Build history of the part. All positions in model axes, mm. A direction names the side the tool comes from. Give positions to 0.01 mm unless a question says otherwise; leave off trailing zeros. Order: outer loops, then holes, each group sorted by start corner. A loop starts at its lowest first (then second) coordinate and runs counter-clockwise, first axis right, second up. Notation, with made-up numbers: (82, 65.5) - (105, 65.5) arc R24 ccw to (105, 89.5) - close; hole circle Ø11 at (54, 16.25). An arc over 180 degrees is marked (long way). Use a Markdown table: item, result.
Autodesk Inventor part; units mm, degrees
ref_plane "YZ Plane" through (0, 0, 0) normal (1, 0, 0) x (0, 1, 0)
ref_plane "XZ Plane" through (0, 0, 0) normal (0, 1, 0) x (-1, 0, 0)
ref_plane "XY Plane" through (0, 0, 0) normal (0, 0, 1) x (1, 0, 0)
sketch "スケッチ1" plane through (0, 0, 0) normal (0, 0, 1) x (1, 0, 0)
  circle A0 centre (0, 0) radius 12.675
  circle A1 centre (0, 0) radius 4
  circle A2 centre (0, 0) radius 10
  circle A3 centre (0, 0) radius 16
  dimension "d0" = 25.35
  dimension "d1" = 8
  dimension "d2" = 20
  dimension "d3" = 32
extrude "押し出し1" add sketch "スケッチ1" along normal blind 3.75 contours A2
extrude "押し出し2" add sketch "スケッチ1" against normal blind 1.7 contours A0
extrude "押し出し3" add sketch "スケッチ1" against normal blind 2.5 contours A2
mirror "ミラー1" about plane through (0, 0, 3.75) normal (0, 0, 1) of "押し出し1", "押し出し2", "押し出し3"
properties part number "timing _pulley_7.5_8"
1) Slice it at D-D (x = 7). Write the cut outline in (y, z), and give its area (3 significant figures).
Computed:
| item | result |
|---|---|
| outline | (-10.57, -1.7) - (-7.14, -1.7) - (-7.14, -2.5) - (7.14, -2.5) - (7.14, -1.7) - (10.57, -1.7) - (10.57, 0) - (7.14, 0) - (7.14, 7.5) - (10.57, 7.5) - (10.57, 9.2) - (7.14, 9.2) - (7.14, 10) - (-7.14, 10) - (-7.14, 9.2) - (-10.57, 9.2) - (-10.57, 7.5) - (-7.14, 7.5) - (-7.14, 0) - (-10.57, 0) - close |
| area | 202 mm² |
2) Wall check: line 1 (Y direction, x = 0, z = 2.25); line 2 (Z direction, x = 4, y = -10.5); line 3 (X direction, y = 1, z = 5). Give the ranges that are in metal, low to high. Write a range as from..to.
Computed:
| item | result |
|---|---|
| line 1 | y = -10..-4, 4..10 |
| line 2 | z = -1.7..0, 7.5..9.2 |
| line 3 | x = -9.95..-3.87, 3.87..9.95 |
3) Tool access for faces 1 (the flat face through (0.9, 10.4, -1.7)), 2 (the flat face through (0.9, 10.4, 0)), 3 (the cylindrical face through (-2.17, 9.76, 9.59)): list every direction of +Z, -Z, +X, -X, +Y, -Y with a clear straight run to the whole face (end or side of a thin tool).
Computed:
| item | result |
|---|---|
| face 1 | -Z |
| face 2 | none |
| face 3 | +Z |
4) Two-plate mould, pull along Z, no slides. Class faces 4 (the cylindrical face through (-2.17, -9.76, -2.09)), 5 (the flat face through (-4.3, 0.1, 10)), 6 (the cylindrical face through (-2.17, 9.76, 3.7)): +Z half, -Z half, draft (parallel to the pull), parting line (faces both ways), or undercut.
Computed:
| item | result |
|---|---|
| face 4 | draft |
| face 5 | +Z half |
| face 6 | undercut |
5) Pin check, flat tips, straight feed: P1, Ø1.5, axis at y = 0.5, z = 4.5, coming from the +X side; P2, Ø3, axis at x = 8, z = 7.5, coming from the +Y side; P3, Ø2, axis at y = 2, z = 6, coming from the -X side. Stop position of each tip, or through.
Computed:
| item | result |
|---|---|
| P1 | stops at x = 10 |
| P2 | stops at y = 10.88 |
| P3 | stops at x = -9.95 |
6) Slice it at C-C (z = 4.75). Write the cut outline in (x, y), and give its area (3 significant figures).
Computed:
| item | result |
|---|---|
| outline | circle Ø20 at (0, 0); hole circle Ø8 at (0, 0) |
| area | 264 mm² |
7) Slice it at A-A (x = 0). Write the cut outline in (y, z) (3 decimals).
Computed:
| item | result |
|---|---|
| outline | (-12.675, -1.7) - (-10, -1.7) - (-10, -2.5) - (-4, -2.5) - (-4, 10) - (-10, 10) - (-10, 9.2) - (-12.675, 9.2) - (-12.675, 7.5) - (-10, 7.5) - (-10, 0) - (-12.675, 0) - close; (4, -2.5) - (10, -2.5) - (10, -1.7) - (12.675, -1.7) - (12.675, 0) - (10, 0) - (10, 7.5) - (12.675, 7.5) - (12.675, 9.2) - (10, 9.2) - (10, 10) - (4, 10) - close |
